Input: part model. Units: mm. Frame: model coordinates. A direction names the side the tool comes from. Give positions to 0.01 mm unless a question says otherwise; leave off trailing zeros. Loops run counter-clockwise (first coordinate to the right, second up) from the corner with the lowest first, then second, coordinate; pieces in that order, holes last.
Autodesk Inventor part; units mm, degrees
ref_plane "YZ Plane" through (0, 0, 0) normal (1, 0, 0) x (0, 1, 0)
ref_plane "XZ Plane" through (0, 0, 0) normal (0, 1, 0) x (-1, 0, 0)
ref_plane "XY Plane" through (0, 0, 0) normal (0, 0, 1) x (1, 0, 0)
sketch "Sketch1" plane through (0, 0, 0) normal (1, 0, 0) x (0, 1, 0)
  circle A0 centre (0, 0) radius 31.75 construction
  line L0 (19.05, -103.6647) -> (-107.95, -103.6647) construction
  line L1 (-107.95, -103.6647) -> (-107.95, -162.179) construction
  line L2 (-107.95, -162.179) -> (19.05, -162.179) construction
  line L3 (19.05, -162.179) -> (19.05, -103.6647) construction
  line L4 (19.05, -103.6647) -> (-107.95, -162.179) construction
  line L5 (-107.95, -103.6647) -> (19.05, -162.179) construction
  line L6 (-25.4, -162.179) -> (-25.4, -365.379) construction
  point P0 (-44.45, -132.9219)
  dimension "d0" = 63.5
  dimension "d2" = 127
  dimension "d3" = 58.5143
  dimension "d4" = 19.05
  dimension "d5" = 162.179
  dimension "d6" = 203.2
  dimension "d7" = 25.4
sketch "Sketch2" plane through (0, 0, 0) normal (1, 0, 0) x (0, 1, 0)
  circle A0 centre (0, 0) radius 31.75 construction
  line L0 (19.05, -103.6647) -> (-107.95, -103.6647) construction
  line L1 (-107.95, -103.6647) -> (-107.95, -162.179) construction
  line L2 (-107.95, -162.179) -> (19.05, -162.179) construction
  line L3 (19.05, -162.179) -> (19.05, -103.6647) construction
  line L4 (19.05, -103.6647) -> (-107.95, -162.179) construction
  line L5 (-107.95, -103.6647) -> (19.05, -162.179) construction
  line L6 (-25.4, -162.179) -> (-25.4, -365.379) construction
  line L7 (-25.0971, -19.4473) -> (25.4, -84.6147)
  line L8 (25.4, -84.6147) -> (25.4, -148.1147)
  line L9 (25.4, -148.1147) -> (-25.4, -200.279)
  line L10 (30.9118, 7.2472) -> (50.8, -77.5826)
  line L11 (50.8, -77.5826) -> (50.8, -179.1826)
  line L12 (50.8, -179.1826) -> (-25.4, -257.429)
  arc A1 (30.9118, 7.2472) -> (-25.0971, -19.4473) centre (0, 0) ccw
  line L13 (6.35, 3.6662) -> (6.35, -3.6662)
  line L14 (6.35, -3.6662) -> (0, -7.3323)
  line L15 (0, -7.3323) -> (-6.35, -3.6662)
  line L16 (-6.35, -3.6662) -> (-6.35, 3.6662)
  line L17 (-6.35, 3.6662) -> (0, 7.3323)
  line L18 (0, 7.3323) -> (6.35, 3.6662)
  line L19 (-25.4, -200.279) -> (-25.4, -257.429)
  point P0 (-44.45, -132.9219)
  point P1 (25.4, -116.3647)
  point P2 (19.05, -132.9219)
  point P3 (-6.35, 0)
  dimension "d8" = 6.35
  dimension "d9" = 63.5
  dimension "d10" = 25.4
  dimension "d11" = 101.6
  dimension "d12" = 12.7
  dimension "d13" = 57.15
  dimension "d28" = 38.1
  dimension "d29" = 19.05
extrude "Extrusion1" add sketch "Sketch2" along normal blind 6.35
sketch "Sketch3" plane through (6.35, 0, 0) normal (1, 0, 0) x (0, 0, -1)
  circle A0 centre (0, 0) radius 25.4 construction
  point P0 (0, 25.4)
  point P1 (-21.997, 12.7)
  point P2 (-21.997, -12.7)
  point P3 (0, -25.4)
  point P4 (21.997, -12.7)
  point P5 (21.997, 12.7)
  dimension "d16" = 50.8
  dimension "d19" = 360
hole "Hole1" at (6.35, 25.4, 0) at (6.35, 12.7, 21.997) at (6.35, -12.7, 21.997) at (6.35, -25.4, 0) at (6.35, -12.7, -21.997) at (6.35, 12.7, -21.997) direction (-1, 0, 0) diameter 5.1054 end through all
sketch "Sketch4" plane through (6.35, 0, 0) normal (1, 0, 0) x (0, 0, -1)
  circle A0 centre (206.629, 25.4) radius 15.875
  line L0 (200.279, -25.4) -> (257.429, -25.4) construction
  point P0 (0, 0)
  dimension "d30" = 31.75
  dimension "d31" = 50.8
  dimension "d32" = 6.35
extrude "Extrusion2" cut sketch "Sketch4" against normal through all
fillet "Fillet1" radius 12.7 2 edges at (3.175, 35.7738, -194.6123) (3.175, 13.6624, -217.3175)
fillet "Fillet2" radius 9.525 6 edges at (3.175, -25.4, -257.429) (3.175, -25.4, -200.279) (3.175, 25.4, -148.1147) (3.175, 50.8, -179.1826) (3.175, 25.4, -84.6147) (3.175, 50.8, -77.5826)
properties part number "CL4-025" material "Aluminum 6061"
(1) Cut plane D-D (z = -84.5). Return the cut outline in (x, y), and give its area (3 significant figures).
Values follow:
outline: (0, 24.78) - (6.35, 24.78) - (6.35, 50.8) - (0, 50.8) - close
area: 165 mm2
(2) Ray query, probe 1 along Y at (x, z) = (4, -23); probe 2 along Y at (x, z) = (3.5, 0); probe 3 along Z at (x, y) = (2, -12.7). Return the intervals inside material, ascending.
Values follow:
probe 1: y = -22.34 to -15.05, -10.35 to 10.35, 15.05 to 38
probe 2: y = -31.75 to -27.95, -22.85 to -6.35, 6.35 to 22.85, 27.95 to 32.61
probe 3: z = -242.98 to -187.24, -35.45 to -24.55, -19.44 to 19.44, 24.55 to 29.1
(3) Mould query, pull axis Z, two halves, no side actions, for faces 1 (the flat face through (3.131, 45.206, -184.926)), 2 (the flat face through (3.131, 40.593, -34.045)), 3 (the flat face through (3.131, 3.131, 5.525)). Classes: +Z half, -Z half, draft (parallel to the pull), parting line (faces both ways), or undercut.
Values follow:
face 1: -Z half
face 2: +Z half
face 3: undercut
(4) Reachability of faces 4 (the flat face through (3, -25.4, -219)), 5 (the cylindrical face through (3.2, 50.1, -178.9)), 6 (the flat face through (3.131, -3.219, 5.474)), 7 (the cylindrical face through (3.22, 24.9, -84.83)) from +Z, -Z, +X, -X, +Y, -Y: full face, straight path, thin tool, end or side. Return the list, or none.
Values follow:
face 4: -Z, +X, -X, -Y
face 5: -Z, +X, -X, +Y
face 6: +X, -X
face 7: +X, -X, -Y
(5) Cut plane B-B (y = -12.7). Return the cut outline in (x, z).
Values follow:
outline: (0, -242.98) - (6.35, -242.98) - (6.35, -187.24) - (0, -187.24) - close; (0, -35.45) - (6.35, -35.45) - (6.35, -24.55) - (0, -24.55) - close; (0, -19.44) - (6.35, -19.44) - (6.35, 19.44) - (0, 19.44) - close; (0, 24.55) - (6.35, 24.55) - (6.35, 29.1) - (0, 29.1) - close
(6) Cut plane A-A (z = 0). Return the cut outline in (x, y), and give its area (3 significant figures).
Values follow:
outline: (0, -31.75) - (6.35, -31.75) - (6.35, -27.95) - (0, -27.95) - close; (0, -22.85) - (6.35, -22.85) - (6.35, -6.35) - (0, -6.35) - close; (0, 6.35) - (6.35, 6.35) - (6.35, 22.85) - (0, 22.85) - close; (0, 27.95) - (6.35, 27.95) - (6.35, 32.61) - (0, 32.61) - close
area: 263 mm2
(7) Cut plane C-C (x = 2.75). Count the separate pieces of the cut face and the enclosed holes in it, and give its area (3 significant figures).
Values follow:
separate pieces: 1
enclosed holes: 7
area: 10,600 mm2
(8) Pin query (flat end, axial travel): pin 1 Ø4 at (y, z) = (23.5, -127) entering from -X; pin 2 Ø4 at (y, z) = (-12.7, 21.997) entering from -X; pin 3 Ø3 at (x, z) = (1.5, -214) entering from -Y; pin 4 Ø1.9 at (x, z) = (2, 1.5) entering from -Y. Return the tip coordinate at first contact, or that it passes through.
Values follow:
pin 1: stops at x = 0
pin 2: passes through
pin 3: stops at y = -25.4
pin 4: stops at y = -31.75
